The drawing under review shows one solid part. Ordinate dimensions are in mm from its lowest x, y, z. Coordinates: 2 decimals unless noted, no trailing zeros. Order: outer loops, then holes, each group sorted by start corner. A loop starts at its lowest first (then second) coordinate and runs counter-clockwise, first axis right, second up. Notation, with made-up numbers: (-37.75, -10.75) - (-29.75, -10.75) arc R25 ccw to (-29.75, 27.25) - close; hole circle Ø7 at (18.25, 5.25). An arc over 180 degrees is marked (long way). Answer in a Markdown table with one row per item.
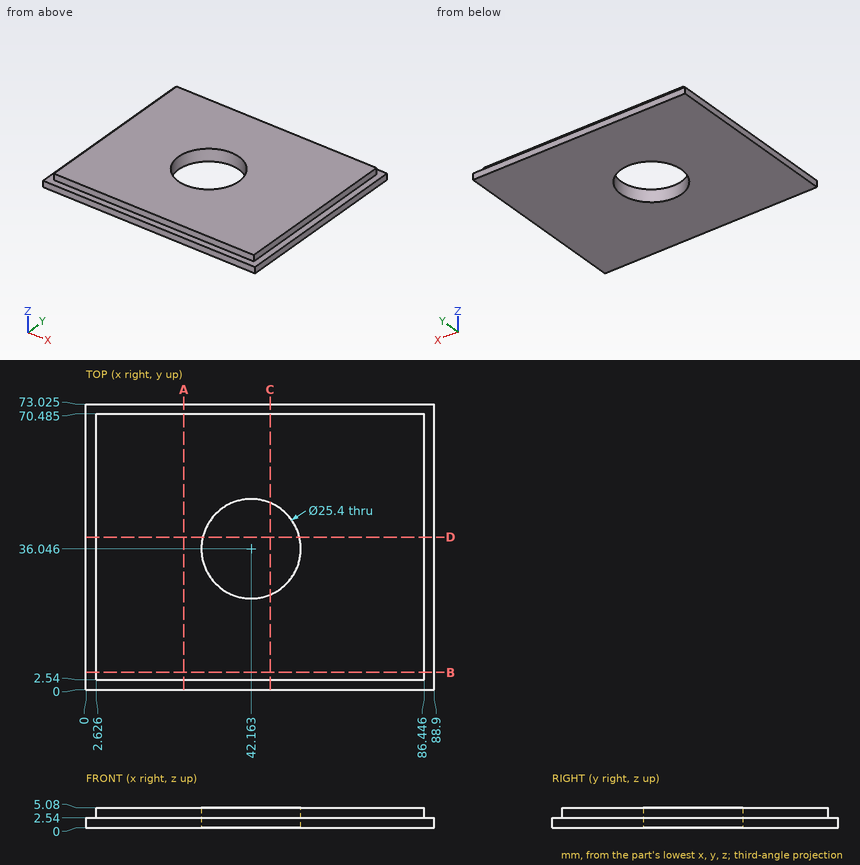
Item 1: We need section A-A, the plane x = 25. Write out the cut boundary in (y, z) (1 decimal).
Check values:
| item | result |
|---|---|
| outline | (0, 0) - (73, 0) - (73, 2.5) - (70.5, 2.5) - (70.5, 5.1) - (2.5, 5.1) - (2.5, 2.5) - (0, 2.5) - close |
Item 2: We need section D-D, the plane y = 39. Write out the cut boundary in (x, z) (1 decimal), then the cut area to 3 significant figures.
Check values:
| item | result |
|---|---|
| outline | (0, 0) - (29.8, 0) - (29.8, 5.1) - (2.6, 5.1) - (2.6, 2.5) - (0, 2.5) - close; (54.5, 0) - (88.9, 0) - (88.9, 2.5) - (86.4, 2.5) - (86.4, 5.1) - (54.5, 5.1) - close |
| area | 313 mm^2 |
Item 3: We need section C-C, the plane x = 47. Write out the cut boundary in (y, z) (1 decimal).
Check values:
| item | result |
|---|---|
| outline | (0, 0) - (24.3, 0) - (24.3, 5.1) - (2.5, 5.1) - (2.5, 2.5) - (0, 2.5) - close; (47.8, 0) - (73, 0) - (73, 2.5) - (70.5, 2.5) - (70.5, 5.1) - (47.8, 5.1) - close |
Item 4: We need section B-B, the plane y = 4.5. Write out the cut boundary in (x, z).
Check values:
| item | result |
|---|---|
| outline | (0, 0) - (88.9, 0) - (88.9, 2.54) - (86.45, 2.54) - (86.45, 5.08) - (2.63, 5.08) - (2.63, 2.54) - (0, 2.54) - close |
Item 5: Clearance check with flat-ended pins moving along their axes: pin 1 Ø2 at (y, z) = (29, 3) entering from -X; pin 2 Ø2 at (x, z) = (20.5, 4) entering from +Y (1 decimal). State where each tip first meets the part, or that it passes through.
Check values:
| item | result |
|---|---|
| pin 1 | x = 0 |
| pin 2 | y = 70.5 |
Item 6: To check wall thickness, follow line 1 (X direction, y = 21, z = 3.3); line 2 (Y direction, x = 25.5, z = 3.35) (1 decimal); line 3 (Y direction, x = 48, z = 4.7) (1 decimal). State the ranges of each line that lie inside material, in increasing order. Write a range as from..to.
Check values:
| item | result |
|---|---|
| line 1 | 2.63..86.45 |
| line 2 | 2.5..70.5 |
| line 3 | 2.5..24.8, 47.3..70.5 |
